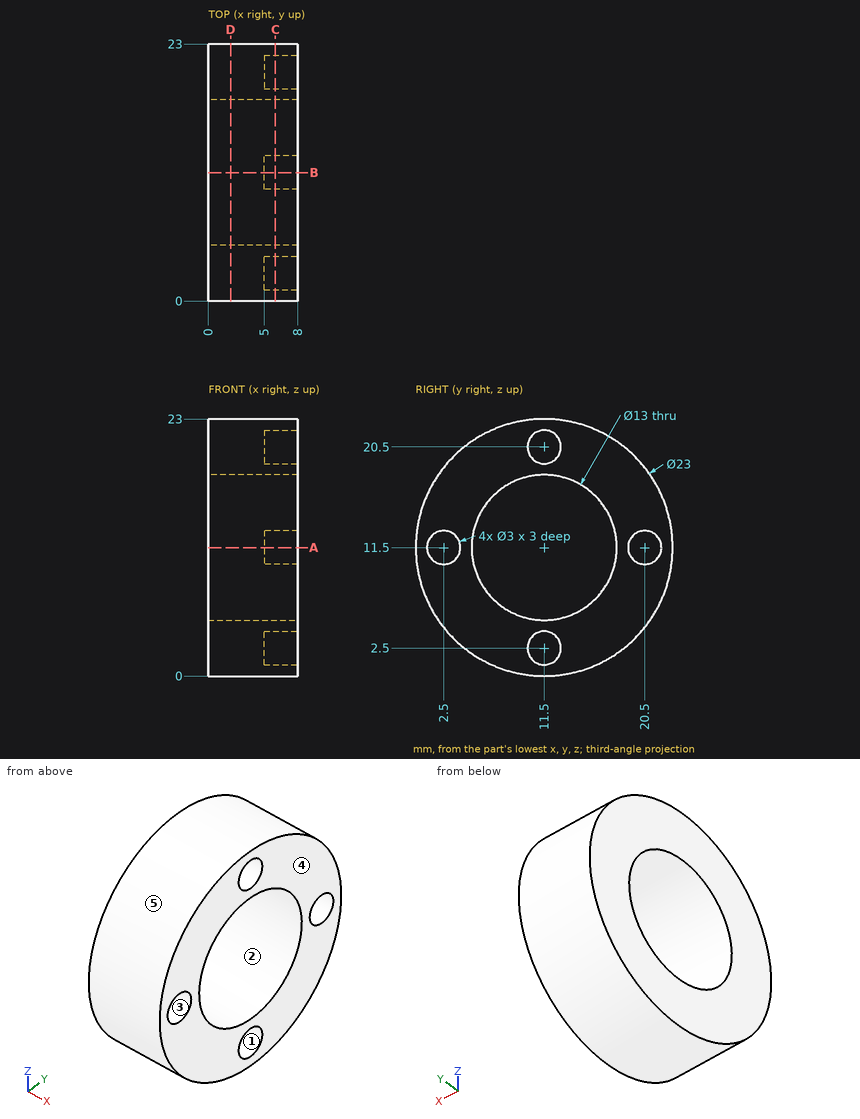
Check sheet for the drawn part. Datum: minimum x, y, z corner. Units: mm. A direction names the side the tool comes from. Give positions to 0.01 mm unless a question says otherwise; leave off trailing zeros. Order: outer loops, then holes, each group sorted by start corner. A loop starts at its lowest first (then second) coordinate and runs counter-clockwise, first axis right, second up. Notation, with made-up numbers: (49, 40.25) -> (78, 40.25) arc R10 cw to (78, 58.25) -> close; hole circle Ø3 at (-31.75, 27). An arc over 180 degrees is marked (long way). One line per item, written item: value.
(1) Sectioned sample at C-C on x = 6. Record the cut outline in (y, z), then the cut area to 3 significant figures.
Final values:
outline: circle Ø23 at (11.5, 11.5); hole circle Ø3 at (2.5, 11.5); hole circle Ø13 at (11.5, 11.5); hole circle Ø3 at (11.5, 2.5); hole circle Ø3 at (11.5, 20.5); hole circle Ø3 at (20.5, 11.5)
area: 254 mm^2
(2) Sectioned sample at D-D on x = 2. Record the cut outline in (y, z), then the cut area to 3 significant figures.
Final values:
outline: circle Ø23 at (11.5, 11.5); hole circle Ø13 at (11.5, 11.5)
area: 283 mm^2
(3) Gauge pin test, flat ends, axial feed: pin 1 (2.5 mm diameter, centred on y = 12, z = 20, fed in from +X); pin 2 (3 mm diameter, centred on x = 2, z = 5.5, fed in from -Y); pin 3 (1.5 mm diameter, centred on x = 5, z = 8.5, fed in from -Y); pin 4 (0.9 mm diameter, centred on y = 3, z = 12, fed in from +X). Record the tip position at first contact, or that the pin passes through.
Final values:
pin 1: x = 8
pin 2: y = 0.92
pin 3: y = 0.22
pin 4: x = 5
(4) Draft check along Z on the marked faces 3, 4 and 5. Enter one of: pulls with the +Z half, pulls with the -Z half, needs draft (parallel to the pull), parting line crosses it, or undercut.
Final values:
face 3: undercut
face 4: needs draft
face 5: parting line crosses it
(5) Tool access check on the marked faces 1 and 2. Record the directions out of +Z, -Z, +X, -X, +Y, -Y that give a thin tool (end or side, any length) a straight path to the whole face; none if there is none.
Final values:
face 1: +X
face 2: +X, -X
(6) Sectioned sample at A-A on z = 11.5. Record the cut outline in (x, y).
Final values:
outline: (0, 0) -> (8, 0) -> (8, 1) -> (5, 1) -> (5, 4) -> (8, 4) -> (8, 5) -> (0, 5) -> close; (0, 18) -> (8, 18) -> (8, 19) -> (5, 19) -> (5, 22) -> (8, 22) -> (8, 23) -> (0, 23) -> close
(7) Scan lines: line 1 along Y through (x, z) = (6.5, 11.5); line 2 along Z through (x, y) = (1, 12.25); line 3 along Y through (x, z) = (7.25, 17.5). Record each from-to range of solid material in increasing order. Write a range as [from, to].
Final values:
line 1: [0, 1], [4, 5], [18, 19], [22, 23]
line 2: [0.02, 5.04], [17.96, 22.98]
line 3: [1.69, 9], [14, 21.31]
